Check sheet for the modelled part. Datum: model origin and axes. Units: mm. Coordinates: 2 decimals unless noted, no trailing zeros. Write each loop counter-clockwise with the first axis right and the second up, starting at its lowest first coordinate (ties: lowest second). Pieces come first, ordered by that corner, then holes. Notation, with made-up numbers: (51, 3.5) - (62, 3.5) arc R27 cw to (62, 21.5) - close; hole circle Ø6 at (-36, 39). An arc over 180 degrees is marked (long way). Use one line per item in the form item = value. Start each with the question number.
1. Cross-section at A-A on x = 1.5. Record the boundary of the cut face in (y, z), then the cut area to 3 significant figures.
2. Scan lines: line 1 along X through (y, z) = (2.5, 3.5); line 2 along Y through (x, z) = (4.5, 25.25); line 3 along Y through (x, z) = (21, 11). Record each from-to range of solid material in increasing order.
3. Cross-section at B-B on y = 18. Record the boundary of the cut face in (x, z).
4. Go/stop test with flat-tipped pins: pin 1 Ø5 at (y, z) = (9.5, 11.5) entering from -X; pin 2 Ø6 at (x, y) = (6, 7) entering from -Z; pin 3 Ø12 at (y, z) = (2.5, 6.5) entering from +X; pin 4 Ø10 at (x, z) = (-13.5, 10) entering from -Y. Record where each tip stops, or that it passes through.
5. Cross-section at D-D on x = -21.5. Record the boundary of the cut face in (y, z).
6. Cross-section at C-C on z = 7. Record the boundary of the cut face in (x, y), then the cut area to 3 significant figures.
```python
from build123d import *

# Parameters (mm, degrees)
BOSS_EXTRUDE2_DEPTH     = 27
CUT_EXTRUDE4_DEPTH      = 37
CUT_EXTRUDE4_DEPTH_BACK = 37
CUT_EXTRUDE5_DEPTH      = 37
CUT_EXTRUDE5_DEPTH_BACK = 37


with BuildPart() as part:
    # Sketch1 → Boss-Extrude2 (new body)
    with BuildSketch(Plane.XY):
        Polygon((15, 0), (-15, 0), (-28.5432741, 21.013798482), (28.5432741, 21.013798482), align=None)
    extrude(amount=BOSS_EXTRUDE2_DEPTH)

    # Sketch3 → Cut-Extrude4 (cut, two sides: drawn at the far end of the back side and taken through both)
    with BuildSketch(Plane(origin=(0, 0, 0), x_dir=(0, 0, -1), z_dir=(1, 0, 0)).offset(-CUT_EXTRUDE4_DEPTH_BACK)):
        Polygon((-13.5, 21.013798482), (0, 0), (0, 21.013798482), align=None)
    extrude(amount=CUT_EXTRUDE4_DEPTH + CUT_EXTRUDE4_DEPTH_BACK, mode=Mode.SUBTRACT)

    # Sketch4 → Cut-Extrude5 (cut, two sides: drawn at the far end of the back side and taken through both)
    with BuildSketch(Plane(origin=(0, 0, 0), x_dir=(0, 0, -1), z_dir=(1, 0, 0)).offset(-CUT_EXTRUDE5_DEPTH_BACK)):
        Polygon((-13.5, 21.013798482), (-27, 0), (-27, 21.013798482), align=None)
    extrude(amount=CUT_EXTRUDE5_DEPTH + CUT_EXTRUDE5_DEPTH_BACK, mode=Mode.SUBTRACT)


solid = part.part
```
Final values:
q1.outline = (0, 0) - (21.01, 13.5) - (0, 27) - close
q1.area = 284 mm²
q2.line_1 = -16.61 to 16.61
q2.line_2 = 0 to 2.72
q2.line_3 = 9.31 to 17.12
q3.outline = (-26.6, 11.56) - (26.6, 11.56) - (26.6, 15.44) - (-26.6, 15.44) - close
q4.pin_1 = -22.73
q4.pin_2 = 2.57
q4.pin_3 = 20.48
q4.pin_4 = 0
q5.outline = (10.09, 6.48) - (21.01, 13.5) - (10.09, 20.52) - close
q6.outline = (-22.02, 10.9) - (-15, 0) - (15, 0) - (22.02, 10.9) - close
q6.area = 403 mm²
